Part model, mm, in its own coordinate system. Round coordinates to 2 decimals unless told otherwise and drop trailing zeros. Loops run counter-clockwise (first coordinate to the right, second up) from the corner with the lowest first, then second, coordinate; pieces in that order, holes last. Notation, with made-up numbers: (-23, 42.25) -> (23, 42.25) arc R29 cw to (23, 63.25) -> close; hole circle Ø4 at (-25, 60.5). An arc over 180 degrees is marked (long way). Answer as a JSON object with one key per item and string values. Group by question number.
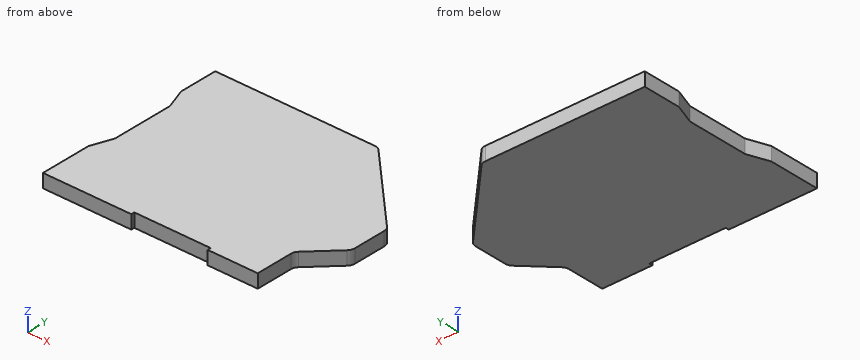
Autodesk Inventor part; units mm, degrees
ref_plane "YZ Plane" through (0, 0, 0) normal (1, 0, 0) x (0, 1, 0)
ref_plane "XZ Plane" through (0, 0, 0) normal (0, 1, 0) x (-1, 0, 0)
ref_plane "XY Plane" through (0, 0, 0) normal (0, 0, 1) x (1, 0, 0)
sketch "Skizze_1" plane through (0, 0, 0) normal (0, 0, 1) x (1, 0, 0)
  line L0 (-20.9, 0) -> (-10.5, 0)
  line L1 (-10.5, 0) -> (-10.5, 0.4)
  line L2 (-10.5, 0.4) -> (-1.5, 0.4)
  line L3 (-1.5, 0.4) -> (-1.5, 0)
  line L4 (-1.5, 0) -> (4.4, 0)
  line L5 (4.4, 0) -> (4.4, 4.3858)
  arc A0 (4.6929, 5.0929) -> (4.4, 4.3858) centre (5.4, 4.3858) ccw
  line L6 (4.6929, 5.0929) -> (7.7071, 8.1071)
  arc A1 (7.7071, 8.1071) -> (8, 8.8142) centre (7, 8.8142) ccw
  line L7 (8, 8.8142) -> (8, 12.6858)
  arc A2 (8, 12.6858) -> (7.7071, 13.3929) centre (7, 12.6858) ccw
  line L8 (7.7071, 13.3929) -> (-1.4071, 22.5071)
  arc A3 (-1.4071, 22.5071) -> (-2.1142, 22.8) centre (-2.1142, 21.8) ccw
  line L9 (-2.1142, 22.8) -> (-20.9, 22.8)
  line L10 (-20.9, 22.8) -> (-20.9, 18.2727)
  line L11 (-20.9, 18.2727) -> (-20, 15.8)
  line L12 (-20, 15.8) -> (-20, 8.5)
  line L13 (-20, 8.5) -> (-20.9, 6.0273)
  line L14 (-20.9, 6.0273) -> (-20.9, 0)
extrude "Extrusion1" add sketch "Skizze_1" along normal blind 1.6
properties part number "745-300"
Item 1: Drop a flat-ended pin along its axis: pin 1 Ø0.8 at (y, z) = (13, 0.5) entering from -X. Give the stop position or say it passes through.
Item 2: Band-saw the part on A-A, the plane z = 1.35. List the corners of the cut face in (x, y), plus the area to 3 significant figures.
Item 3: Band-saw the part on C-C, the plane x = 1.5. List the corners of the cut face in (y, z).
Item 4: Band-saw the part on B-B, the plane y = 10.75. List the corners of the cut face in (x, z), plus the area to 3 significant figures.
Item 5: Drill centre lines: line 1 (X direction, y = 4.5, z = 1.1); line 2 (Y direction, x = -7.5, z = 0.2); line 3 (X direction, y = 10.75, z = 1.25). Where is each one in solid material? Low to high.
Entries:
{
 "1": {"pin 1": "x = -20"},
 "2": {"outline": "(-20.9, 0) -> (-10.5, 0) -> (-10.5, 0.4) -> (-1.5, 0.4) -> (-1.5, 0) -> (4.4, 0) -> (4.4, 4.39) arc R1 cw to (4.69, 5.09) -> (7.71, 8.11) arc R1 ccw to (8, 8.81) -> (8, 12.69) arc R1 ccw to (7.71, 13.39) -> (-1.41, 22.51) arc R1 ccw to (-2.11, 22.8) -> (-20.9, 22.8) -> (-20.9, 18.27) -> (-20, 15.8) -> (-20, 8.5) -> (-20.9, 6.03) -> close", "area": "576 mm²"},
 "3": {"outline": "(0, 0) -> (19.6, 0) -> (19.6, 1.6) -> (0, 1.6) -> close"},
 "4": {"outline": "(-20, 0) -> (8, 0) -> (8, 1.6) -> (-20, 1.6) -> close", "area": "44.8 mm²"},
 "5": {"line 1": "-20.9 to 4.41", "line 2": "0.4 to 22.8", "line 3": "-20 to 8"}
}
